Part print with two shaded views. Sizes in mm from the minimum x, y, z corner. Give positions to 0.01 mm unless a question says otherwise; leave off trailing zeros. Write each loop counter-clockwise with the first axis right and the second up, starting at its lowest first coordinate (ties: lowest second). Pieces come first, ordered by that corner, then holes. Notation, with made-up numbers: (12, 13.25) - (39, 13.25) arc R21 ccw to (39, 17.25) - close; hole circle Ø2 at (3.25, 44.25). An arc over 180 degrees is marked (long way). One line per item, written item: value. Start each with the question number.
(1) Cut at B-B, the plane x = 0.75. List the corners of the cut face in (y, z).
(2) Cut at A-A, the plane z = 2. List the corners of the cut face in (x, y), and give its area (3 significant figures).
(3) Probe L1, parallel to Y at x = 4.5, z = 6; L2, parallel to Z at x = 1, y = 7.5; L3, parallel to X at y = 8.5, z = 2 (1 decimal). List the from-to ranges inside material, lowest first.
(4) Cut at D-D, the plane y = 1.5. List the corners of the cut face in (x, z), and give its area (3 significant figures).
(5) Cut at C-C, the plane z = 13.25. List the corners of the cut face in (x, y).
(6) Mould opens along Y. For the marked faces 1, 2, 3 and 4 say: pulls with the +Y half, pulls with the -Y half, needs draft (parallel to the pull), parting line crosses it, or undercut.
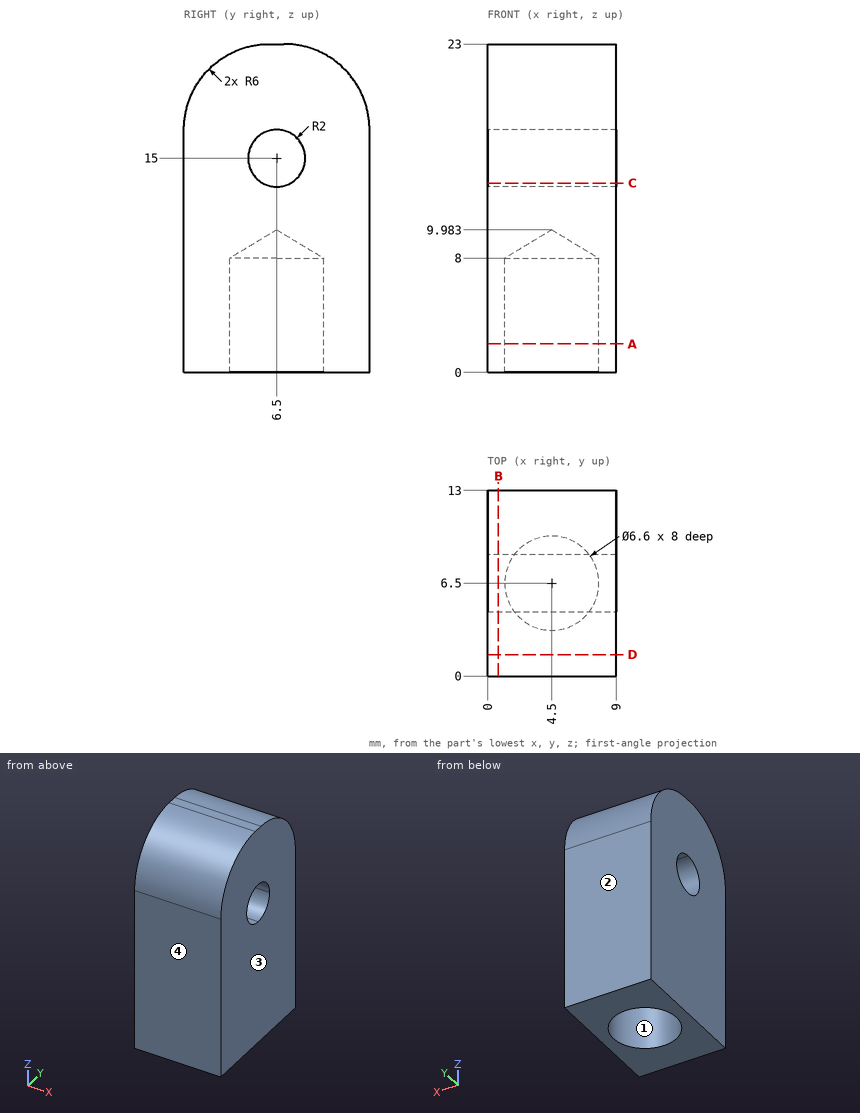
Answers follow:
1. outline: (0, 0) - (13, 0) - (13, 17) arc R6 ccw to (7, 23) - (6, 23) arc R6 ccw to (0, 17) - close; hole circle Ø4 at (6.5, 15)
2. outline: (0, 0) - (9, 0) - (9, 13) - (0, 13) - close; hole circle Ø6.6 at (4.5, 6.5)
2. area: 82.8 mm²
3. L1: y = 0 to 3.2, 9.8 to 13
3. L2: z = 0 to 13.27, 16.73 to 22.98
3. L3: x = 0 to 1.9, 7.1 to 9
4. outline: (0, 0) - (9, 0) - (9, 20.97) - (0, 20.97) - close
4. area: 189 mm²
5. outline: (0, 0) - (9, 0) - (9, 5.53) - (0, 5.53) - close; (0, 7.47) - (9, 7.47) - (9, 13) - (0, 13) - close
6. face 1: undercut
6. face 2: pulls with the +Y half
6. face 3: needs draft
6. face 4: pulls with the -Y half
